Input: dimensioned drawing with shaded views. Units: mm. Origin: part minimum x, y, z. A direction names the side the tool comes from. Round coordinates to 2 decimals unless told otherwise and drop trailing zeros. Order: outer loops, then holes, each group sorted by start corner. A loop starts at its lowest first (then second) coordinate and runs counter-clockwise, first axis right, second up. Notation, with made-up numbers: M 62,5 L 118,5 A27 cw 118,26 Z; hole C -38,-38.5 d11. An arc over 180 degrees is marked long. Answer as CSV lines item,"result". Start each with the question number.
Item 1: Section query A-A on x = 1430. Return the cut outline in (y, z), plus the area to 3 significant figures.
Item 2: Line query: line 1 (Z direction, x = 577, y = 924); line 2 (Z direction, x = 1249, y = 1154); line 3 (X direction, y = 649, z = 1147). Output: solid intervals per line, ascending. Write a range as [from, to].
Item 3: Set-up query: the marked faces 1, 2, 3, 4 and 5. Return all of +Z, -Z, +X, -X, +Y, -Y with unobstructed straight access to the full face (end or side cutting, diameter ignored); none if empty.
Item 4: First-contact query: P1, Ø2, axis at x = 349, z = 753, coming from the -Y side. Flat tip, straight axial feed; report the tip coordinate or a pass-through.
Item 5: Section query C-C on y = 527. Return the cut outline in (x, z), plus the area to 3 significant figures.
Item 6: Section query B-B on z = 910. Return the cut outline in (x, y).
Item 7: Section query D-D on x = 138.5. Return the cut outline in (y, z).
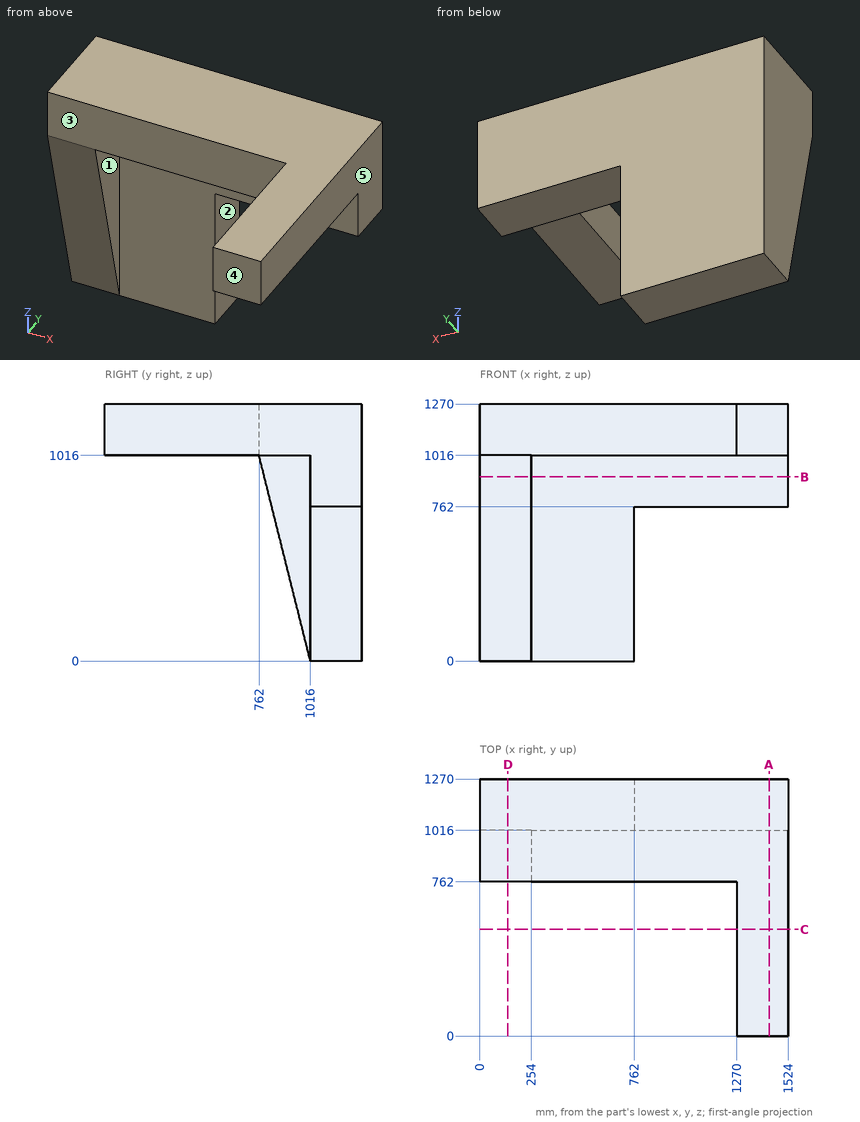
Results:
1,outline,"M 0,1016 L 1016,1016 L 1016,762 L 1270,762 L 1270,1270 L 0,1270 Z"
1,area,"387,000 mm^2"
2,line 1,"[1016, 1270]"
2,line 2,"[762, 1270]"
2,line 3,"[1270, 1524]"
3,face 1,"-Z, +X, -Y"
3,face 2,"-Z, +X, +Y, -Y"
3,face 3,"+Z, -Z, -X, -Y"
3,face 4,"+Z, -Z, +X, -X, -Y"
3,face 5,"+Z, -Z, +X, +Y, -Y"
4,P1,"y = 1016"
5,outline,"M 1270,1016 L 1524,1016 L 1524,1270 L 1270,1270 Z"
5,area,"64,500 mm^2"
6,outline,"M 0,788.5 L 254,788.5 L 254,1016 L 1524,1016 L 1524,1270 L 0,1270 Z"
7,outline,"M 762,1016 L 1016,0 L 1270,0 L 1270,1270 L 762,1270 Z"
